from build123d import *

# Parameters (mm, degrees)
CROQUIS2_W              = 450
CROQUIS2_H              = 90
SALIENTE_EXTRUIR1_DEPTH = 10
CROQUIS6_R              = 18
CROQUIS6_R_2            = 2
CORTAR_EXTRUIR1_DEPTH   = 460.020696701
CHAFL_N5_SIZE           = 0.5
CROQUIS9_R              = 10
CROQUIS9_R_2            = 3.5
CORTAR_EXTRUIR2_DEPTH   = 460.020696701
CHAFL_N6_SIZE           = 0.5


with BuildPart() as part:
    # Croquis2 → Saliente-Extruir1 (new body)
    with BuildSketch(Plane.XY):
        with Locations((225, 45)):
            Rectangle(CROQUIS2_W, CROQUIS2_H)
    extrude(amount=SALIENTE_EXTRUIR1_DEPTH)

    # Croquis6 → Cortar-Extruir1 (cut, through all)
    with BuildSketch(Plane.XY.offset(10)):
        with Locations((225, 58)):
            Circle(CROQUIS6_R)
        with Locations((209.437767177, 73.550463323)):
            Circle(CROQUIS6_R_2)
        with Locations((240.550463323, 73.562232823)):
            Circle(CROQUIS6_R_2)
        with Locations((240.562232823, 42.449536677)):
            Circle(CROQUIS6_R_2)
        with Locations((209.449536677, 42.437767177)):
            Circle(CROQUIS6_R_2)
    extrude(amount=-CORTAR_EXTRUIR1_DEPTH, mode=Mode.SUBTRACT)

    # Chaflán5
    chafl_n5_edges = [part.edges().sort_by_distance(p)[0] for p in [
        (207, 58, 0),
        (207, 58, 10),
        (207.437767177, 73.550463323, 0),
        (207.437767177, 73.550463323, 10),
        (238.550463323, 73.562232823, 0),
        (238.550463323, 73.562232823, 10),
        (238.562232823, 42.449536677, 0),
        (238.562232823, 42.449536677, 10),
        (207.449536677, 42.437767177, 0),
        (207.449536677, 42.437767177, 10),
    ]]
    chamfer(chafl_n5_edges, length=CHAFL_N5_SIZE)

    # Croquis9 → Cortar-Extruir2 (cut, through all)
    with BuildSketch(Plane.XY.offset(10)):
        with Locations((50, 50)):
            Circle(CROQUIS9_R)
        with Locations(Location((400, 50, 0), (0, 0, 180))):
            Circle(CROQUIS9_R)
        with Locations((26, 50)):
            Circle(CROQUIS9_R_2)
        with Locations((74, 50)):
            Circle(CROQUIS9_R_2)
        with Locations(Location((376, 50, 0), (0, 0, 180))):
            Circle(CROQUIS9_R_2)
        with Locations(Location((424, 50, 0), (0, 0, 180))):
            Circle(CROQUIS9_R_2)
    extrude(amount=-CORTAR_EXTRUIR2_DEPTH, mode=Mode.SUBTRACT)

    # Chaflán6
    chafl_n6_edges = [part.edges().sort_by_distance(p)[0] for p in [
        (40, 50, 0),
        (40, 50, 10),
        (410, 50, 0),
        (410, 50, 10),
        (22.5, 50, 0),
        (22.5, 50, 10),
        (70.5, 50, 0),
        (70.5, 50, 10),
        (379.5, 50, 0),
        (379.5, 50, 10),
        (427.5, 50, 0),
        (427.5, 50, 10),
    ]]
    chamfer(chafl_n6_edges, length=CHAFL_N6_SIZE)


solid = part.part
CAD build for the part. Positions are in the model's coordinates, mm. Give positions to 0.01 mm unless a question says otherwise; leave off trailing zeros. Order: outer loops, then holes, each group sorted by start corner. A loop starts at its lowest first (then second) coordinate and runs counter-clockwise, first axis right, second up. Notation, with made-up numbers: (11.25, -34) - (32.25, -34) arc R3 cw to (32.25, -29) - close; hole circle Ø11 at (6.25, 13.25). An arc over 180 degrees is marked (long way). Write each question's results on one line, items separated by ' | '.
1. Probe L1, parallel to Y at x = 26, z = 5; L2, parallel to X at y = 41.5, z = 2.25; L3, parallel to X at y = 43, z = 5.5. List the from-to ranges inside material, lowest first. Write a range as from..to.
Calculated:
L1: y = 0..46.5, 53.5..90 | L2: x = 0..44.73, 55.27..207.68, 211.22..217.81, 232.19..238.8, 242.32..394.73, 405.27..450 | L3: x = 0..42.86, 57.14..207.53, 211.37..215.05, 234.95..238.64, 242.48..392.86, 407.14..450
2. Saw through at B-B on z = 2. Count the separate pieces of the cut face and the enclosed holes in it, and give its area (3 significant figures).
Calculated:
separate pieces: 1 | enclosed holes: 11 | area: 38,600 mm2
3. Saw through at A-A on x = 50. List the corners of the cut face in (y, z), and give its area (4 significant figures).
Calculated:
outline: (0, 0) - (39.5, 0) - (40, 0.5) - (40, 9.5) - (39.5, 10) - (0, 10) - close; (60, 0.5) - (60.5, 0) - (90, 0) - (90, 10) - (60.5, 10) - (60, 9.5) - close | area: 699.5 mm2
4. Pull direction Y, two halves, no side cores. Call faces 1 (the face through (222, 0, 5)), 2 (the face through (25.54, 53.47, 5.06)), 3 (the face through (0, 44, 5)): released by +Y, released by -Y, zero draft, split by the parting line, or undercut.
Calculated:
face 1: released by -Y | face 2: undercut | face 3: zero draft
